Here's how the part is built. I have some questions about the finished solid (model axes, mm). A direction names the side the tool comes from. Coordinates: 2 decimals unless noted, no trailing zeros. Write each loop counter-clockwise with the first axis right and the second up, starting at its lowest first coordinate (ties: lowest second). Pieces come first, ordered by that corner, then holes.
Autodesk Inventor part; units mm, degrees
ref_plane "YZ Plane" through (0, 0, 0) normal (1, 0, 0) x (0, 1, 0)
ref_plane "XZ Plane" through (0, 0, 0) normal (0, 1, 0) x (-1, 0, 0)
ref_plane "XY Plane" through (0, 0, 0) normal (0, 0, 1) x (1, 0, 0)
sketch "草图1" plane through (0, 0, 0) normal (0, 0, 1) x (1, 0, 0)
  circle A0 centre (0, 0) radius 18.5
  dimension "d0" = 37
extrude "拉伸1" add sketch "草图1" along normal blind 22
sketch "草图2" plane through (0, 0, 22) normal (0, 0, 1) x (1, 0, 0)
  circle A0 centre (0, 0) radius 17
  dimension "d3" = 34
extrude "拉伸2" add sketch "草图2" along normal blind 33.5
chamfer "倒角1" distance 2 angle 45 1 edges at (-17, 0, 55.5)
sketch "草图3" plane through (0, 0, 0) normal (0, 0, -1) x (-1, 0, 0)
  circle A0 centre (7, 0) radius 5
  line L0 (33.5538, 0) -> (-37.1398, 0)
  point P0 (0, 0)
  dimension "d9" = 10
  dimension "d10" = 7
extrude "拉伸3" add sketch "草图3" along normal blind 6
sketch "草图4" plane through (-7, 0, -6) normal (0, 0, -1) x (-1, 0, 0)
  circle A0 centre (0, 0) radius 5
  circle A1 centre (0, 0) radius 3
  point P0 (-7, 0)
  dimension "d13" = 6
extrude "拉伸4" add sketch "草图4" along normal blind 15.5 contours A1
chamfer "倒角2" distance 0.5 angle 45 1 edges at (-2, 0, -6)
sketch "草图5" plane through (0, 0, 0) normal (0, 0, -1) x (-1, 0, 0)
  circle A0 centre (7, 0) radius 5
  circle A1 centre (7, 0) radius 7
  circle A2 centre (0, 0) radius 11
  point P0 (8.6429, -6.8045)
  point P1 (8.6429, 6.8045)
  dimension "d19" = 22
extrude "拉伸5" cut sketch "草图5" against normal blind 1 contours A1 A2
chamfer "倒角3" distance 1 angle 45 2 edges at (11, 0, 0) (-18.5, 0, 0)
sketch "草图6" plane through (0, 0, 0) normal (0, 0, -1) x (-1, 0, 0)
  circle A0 centre (0, 0) radius 15.5 construction
  circle A1 centre (0, 15.5) radius 1.6
  line L0 (0, 15.5) -> (0, 0) construction
  arc A2 (10.2857, 6.1809) -> (10.2857, -6.1809) centre (7, 0) ccw
  circle A3 centre (-13.4234, 7.75) radius 1.6
  circle A4 centre (-13.4234, -7.75) radius 1.6
  circle A5 centre (0, -15.5) radius 1.6
  circle A6 centre (13.4234, -7.75) radius 1.6
  circle A7 centre (13.4234, 7.75) radius 1.6
  dimension "d25" = 31
  dimension "d26" = 3.2
  dimension "d29" = 360
extrude "拉伸6" cut sketch "草图6" against normal blind 10
properties part number "JGB37-520"
1) Imagine slicing it at B-B on z = 47.5. Please give me the cut outline in (x, y), then the cut area to 3 significant figures.
Values follow:
outline: circle Ø34 at (0, 0)
area: 908 mm2
2) We'd pull the mould along Y, two halves only. Please class faces 4 (the face through (-7, 0, -21.5)), 5 (the face through (-13, -8, 10)), 6 (the face through (9.139, -14.334, 37.53)): pulls with the +Y half, pulls with the -Y half, needs draft (parallel to the pull), parting line crosses it, or undercut.
Values follow:
face 4: needs draft
face 5: undercut
face 6: parting line crosses it
3) I need wall thicknesses on probe 1 along Y at (x, z) = (0, 8); probe 2 along X at (y, z) = (7, 4); probe 3 along Z at (x, y) = (-7.5, -6). Which ranges of each line are inside material? Lowest first, please.
Values follow:
probe 1: y = -18.5 to -17.1, -13.9 to 13.9, 17.1 to 18.5
probe 2: x = -17.12 to -14.84, -12.01 to 12.01, 14.84 to 17.12
probe 3: z = 0 to 55.5
4) On a 3-axis mill with a long thin cutter (end or side, diameter ignored), from which of +Z, -Z, +X, -X, +Y, -Y can I reach the whole of each face in a straight line? I mean faces 1 (the face through (5.4, -16.4, 22)), 2 (the face through (-4.01, 18.06, 11.35)), 3 (the face through (13, 8, 10)). Say none if no direction works.
Values follow:
face 1: +Z
face 2: +Z, -Z
face 3: -Z
5) Will these pins go through, and if not, where does the flat tip stop? pin 1 (2.5 mm diameter, centred on x = -13.42, y = 7.75, fed in from +Z); pin 2 (3 mm diameter, centred on x = 13.42, y = 7.75, fed in from -Z); pin 3 (10 mm diameter, centred on x = 5.5, z = 37.5, fed in from -Y); pin 4 (1 mm diameter, centred on x = -4, z = 18.5, fed in from +Y).
Values follow:
pin 1: stops at z = 55.5
pin 2: stops at z = 10
pin 3: stops at y = -16.99
pin 4: stops at y = 18.17
6) Imagine slicing it at A-A on y = 0. Please give me the cut outline in (x, z), then the cut area to 3 significant figures.
Values follow:
outline: (-18.5, 1) - (-17.5, 0) - (-12, 0) - (-12, -5.5) - (-11.5, -6) - (-10, -6) - (-10, -21.5) - (-4, -21.5) - (-4, -6) - (-2.5, -6) - (-2, -5.5) - (-2, 0) - (0, 0) - (0, 1) - (11, 1) - (12, 0) - (17.5, 0) - (18.5, 1) - (18.5, 22) - (17, 22) - (17, 53.5) - (15, 55.5) - (-15, 55.5) - (-17, 53.5) - (-17, 22) - (-18.5, 22) - close
area: 2,090 mm2
